Model file for the job. Use its own axes, mm. Face numbers are marked on the shaded views. Give positions to 0.01 mm unless a question says otherwise; leave off trailing zeros. Write each loop counter-clockwise with the first axis right and the second up, starting at its lowest first coordinate (ties: lowest second). Pieces come first, ordered by that corner, then holes.
```python
from build123d import *

# Parameters (mm, degrees)
SKETCH1_R                       = 11.938
EXTRUDE1_DEPTH                  = 1.9812
SKETCH2_R                       = 4.445
EXTRUDE2_DEPTH                  = 2.286
F_3_64_0_04688_DIAMETER_HOLE1_D = 1.190752
CIRPATTERN1_COUNT               = 2
SKETCH6_R                       = 3.7465
SKETCH6_R_2                     = 3.0353
EXTRUDE4_DEPTH                  = 0.508
EXTRUDE3_DEPTH                  = 0.508


with BuildPart() as part:
    # Sketch1 → Extrude1 (new body)
    with BuildSketch(Plane(origin=(0, 0, 0), x_dir=(1, 0, 0), z_dir=(0, 1, 0))):
        Circle(SKETCH1_R)
    extrude(amount=-EXTRUDE1_DEPTH)

    # Sketch2 → Extrude2 (add)
    with BuildSketch(Plane.XZ.offset(1.9812)):
        Circle(SKETCH2_R)
    extrude(amount=EXTRUDE2_DEPTH)

    # 3/64 (0.04688) Diameter Hole1 (through all)
    with Locations(Plane(origin=(0, 0, -6.858), x_dir=(0, 0, 1), z_dir=(0, 1, 0))):
        with Locations((0, 0), (0.413588007, -2.345574143), (0.413588007, 2.345574143), (-2.331254139, 3.344614982), (-2.921, 0), (-2.331254139, -3.344614982), (3.991187159, -7.876503547), (6.858, -8.382), (9.724812841, -7.876503547)):
            f_3_64_0_04688_diameter_hole1 = Hole(F_3_64_0_04688_DIAMETER_HOLE1_D / 2)

    # CirPattern1: 3/64 (0.04688) Diameter Hole1 ×2 about axis
    cirpattern1_axis = Axis((0, 0, 0), (0, 1, 0))
    for i in range(1, CIRPATTERN1_COUNT):
        add(f_3_64_0_04688_diameter_hole1.rotate(cirpattern1_axis, i * 360 / CIRPATTERN1_COUNT), mode=Mode.SUBTRACT)

    # Sketch6 → Extrude4 (add)
    with BuildSketch(Plane(origin=(0, 0, 0), x_dir=(1, 0, 0), z_dir=(0, 1, 0))):
        Circle(SKETCH6_R)
        Circle(SKETCH6_R_2, mode=Mode.SUBTRACT)
    extrude(amount=EXTRUDE4_DEPTH)

    # Sketch5 → Extrude3 (add)
    with BuildSketch(Plane(origin=(0, 0, 0), x_dir=(1, 0, 0), z_dir=(0, 1, 0))):
        Polygon((-2.72405404, 9.39824726), (0, 11.684), (2.72405404, 9.39824726), (2.234249881, 8.814521394), (1.524, 9.410491808), (1.524, 4.572), (-1.524, 4.572), (-1.524, 9.410491808), (-2.234249881, 8.814521394), align=None)
        Polygon((0, 10.689279646), (-0.889, 9.943320073), (-0.889, 5.207), (0.889, 5.207), (0.889, 9.943320073), align=None, mode=Mode.SUBTRACT)
    extrude(amount=EXTRUDE3_DEPTH)


solid = part.part
```
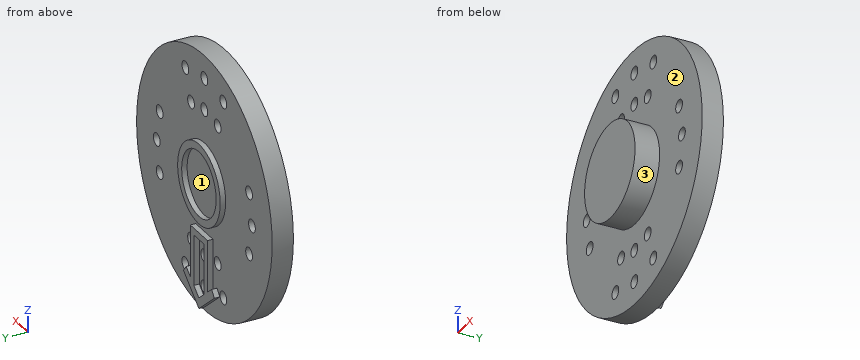
1. Pin check, flat tips, straight feed: P1, Ø0.6, axis at y = 0.5, z = -7, coming from the -X side; P2, Ø4, axis at x = 8, z = -5, coming from the +Y side; P3, Ø4, axis at x = 5.5, z = 6.5, coming from the -Y side. Stop position of each tip, or through.
Calculated:
P1: stops at x = -1.52
P2: stops at y = 0
P3: stops at y = -1.98
2. Slice it at C-C, the plane y = -3.6. Write the cut outline in (x, z) (3 decimals).
Calculated:
outline: circle Ø8.89 at (0, 0)
3. Slice it at A-A, the plane z = 0. Write the cut outline in (x, y) (1 decimal), and give its area (3 significant figures).
Calculated:
outline: (-11.9, -2) - (-9, -2) - (-9, 0) - (-11.9, 0) - close; (-7.8, -2) - (-4.4, -2) - (-4.4, -4.3) - (4.4, -4.3) - (4.4, -2) - (7.8, -2) - (7.8, 0) - (3.7, 0) - (3.7, 0.5) - (3, 0.5) - (3, 0) - (-3, 0) - (-3, 0.5) - (-3.7, 0.5) - (-3.7, 0) - (-7.8, 0) - close; (9, -2) - (11.9, -2) - (11.9, 0) - (9, 0) - close
area: 63.6 mm2
4. Pull direction Z, two halves, no side cores. Call the marked faces 1, 2 and 3: +Z half, -Z half, draft (parallel to the pull), parting line (faces both ways), or undercut.
Calculated:
face 1: undercut
face 2: draft
face 3: parting line
5. Slice it at B-B, the plane y = -1.6. State how many separate pieces and enclosed holes the cut face has, and give its area (3 significant figures).
Calculated:
separate pieces: 1
enclosed holes: 18
area: 428 mm2
6. Slice it at D-D, the plane x = 6.75. Write the cut outline in (y, z).
Calculated:
outline: (-1.98, -9.85) - (0, -9.85) - (0, 9.85) - (-1.98, 9.85) - close
7. Probe probe 1 along X at (y, z) = (-0.5, 0); probe 2 along Z at (x, y) = (3.25, -0.3); probe 3 along X at (y, z) = (0.15, -6). List the from-to ranges inside material, lowest first.
Calculated:
probe 1: x = -11.94 to -8.98, -7.79 to 7.79, 8.98 to 11.94
probe 2: z = -11.49 to -9.78, -8.6 to 8.6, 9.78 to 11.49
probe 3: x = -1.52 to -0.89, 0.89 to 1.52
